Geometry: final body of the model. Coordinates: model frame, mm. A direction names the side the tool comes from. Coordinates: 2 decimals unless noted, no trailing zeros. Loops run counter-clockwise (first coordinate to the right, second up) from the corner with the lowest first, then second, coordinate; pieces in that order, holes last. Notation, with made-up numbers: (-31, 76.25) - (-11, 76.25) arc R14 cw to (-11, 82.25) - close; hole circle Ø1 at (-31.5, 79). An arc over 180 degrees is marked (long way). Answer in a Markdown table with one row per item.
from build123d import *

# Parameters (mm, degrees)
SKETCH1_W                                  = 115
SKETCH1_H                                  = 115
BOSS_EXTRUDE1_DEPTH                        = 40
FILLET1_R                                  = 10
SKETCH4_W                                  = 101
SKETCH4_H                                  = 101
CUT_EXTRUDE3_DEPTH                         = 40
SKETCH7_W                                  = 90
SKETCH7_H                                  = 90
CUT_EXTRUDE5_DEPTH                         = 60
FILLET3_R                                  = 10
SKETCH8_R                                  = 3.15
CUT_EXTRUDE6_DEPTH                         = 35
MIRROR2_AT_THE_SECOND_PLANE_COPY_1_SKETC_R = 3.15
MIRROR2_AT_THE_SECOND_PLANE_COPY_1_DEPTH   = 35
SKETCH9_R                                  = 1.25
CUT_EXTRUDE7_DEPTH                         = 15
MIRROR3_AT_THE_SECOND_PLANE_COPY_1_SKETC_R = 1.25
MIRROR3_AT_THE_SECOND_PLANE_COPY_1_DEPTH   = 15
SKETCH10_R                                 = 2.5
CUT_EXTRUDE8_DEPTH                         = 3
MIRROR4_AT_THE_SECOND_PLANE_COPY_1_SKETC_R = 2.5
MIRROR4_AT_THE_SECOND_PLANE_COPY_1_DEPTH   = 3
SKETCH11_W                                 = 40
SKETCH11_H                                 = 90
CUT_EXTRUDE9_DEPTH                         = 11
SKETCH13_W                                 = 2.5
SKETCH13_H                                 = 90
BOSS_EXTRUDE2_DEPTH                        = 17
FILLET6_R                                  = 2
SKETCH14_W                                 = 20
SKETCH14_H                                 = 30
CUT_EXTRUDE10_DEPTH                        = 11
SKETCH15_W                                 = 10
SKETCH15_H                                 = 2.5
BOSS_EXTRUDE3_DEPTH                        = 19
FILLET7_R                                  = 2
SKETCH16_W                                 = 115
SKETCH16_H                                 = 115
CUT_EXTRUDE12_DEPTH                        = 20
SKETCH17_W                                 = 10
SKETCH17_H                                 = 80
CUT_EXTRUDE13_DEPTH                        = 15
SKETCH20_R                                 = 2.25
CUT_EXTRUDE14_DEPTH                        = 25
MIRROR8_AT_THE_SECOND_PLANE_COPY_1_SKETC_R = 2.25
MIRROR8_AT_THE_SECOND_PLANE_COPY_1_DEPTH   = 25
SKETCH21_R                                 = 1.75
CUT_EXTRUDE15_DEPTH                        = 20
MIRROR9_AT_THE_SECOND_PLANE_COPY_1_SKETC_R = 1.75
MIRROR9_AT_THE_SECOND_PLANE_COPY_1_DEPTH   = 20
SKETCH24_W                                 = 15
SKETCH24_H                                 = 30
CUT_EXTRUDE16_DEPTH                        = 10
MIRROR10_AT_THE_SECOND_PLANE_COPY_1_SKET_W = 15
MIRROR10_AT_THE_SECOND_PLANE_COPY_1_SKET_H = 30
MIRROR10_AT_THE_SECOND_PLANE_COPY_1_DEPTH  = 10
SKETCH25_R                                 = 4
CUT_EXTRUDE17_DEPTH                        = 7.5
MIRROR11_AT_THE_SECOND_PLANE_COPY_1_SKET_R = 4
MIRROR11_AT_THE_SECOND_PLANE_COPY_1_DEPTH  = 7.5


with BuildPart() as part:
    # Sketch1 → Boss-Extrude1 (new, symmetric)
    with BuildSketch(Plane.XY):
        Rectangle(SKETCH1_W, SKETCH1_H)
    extrude(amount=BOSS_EXTRUDE1_DEPTH, both=True)

    # Fillet1
    fillet1_edges = [part.edges().sort_by_distance(p)[0] for p in [
        (-57.5, 57.5, 0),
        (57.5, 57.5, 0),
        (57.5, -57.5, 0),
        (-57.5, -57.5, 0),
    ]]
    fillet(fillet1_edges, radius=FILLET1_R)

    # Sketch4 → Cut-Extrude3 (cut)
    with BuildSketch(Plane.XY.offset(40)):
        Rectangle(SKETCH4_W, SKETCH4_H)
    extrude(amount=-CUT_EXTRUDE3_DEPTH, mode=Mode.SUBTRACT)

    # Sketch7 → Cut-Extrude5 (cut)
    with BuildSketch(Plane.XY):
        Rectangle(SKETCH7_W, SKETCH7_H)
    extrude(amount=-CUT_EXTRUDE5_DEPTH, mode=Mode.SUBTRACT)

    # Fillet3
    fillet3_edges = [part.edges().sort_by_distance(p)[0] for p in [
        (-45, -45, -20),
        (-45, 45, -20),
        (45, 45, -20),
        (45, -45, -20),
    ]]
    fillet(fillet3_edges, radius=FILLET3_R)

    # Sketch8 → Cut-Extrude6 (cut)
    with BuildSketch(Plane(origin=(0, 0, -40), x_dir=(-1, 0, 0), z_dir=(0, 0, -1))):
        with Locations((-48, 48)):
            Circle(SKETCH8_R)
    cut_extrude6 = extrude(amount=-CUT_EXTRUDE6_DEPTH, mode=Mode.SUBTRACT)

    # Mirror2: Cut-Extrude6 across plane
    add(cut_extrude6.mirror(Plane.ZX), mode=Mode.SUBTRACT)

    # Mirror2 at the second plane: Cut-Extrude6 across plane
    add(cut_extrude6.mirror(Plane(origin=(0, 0, 0), x_dir=(0, 0, 1), z_dir=(1, 0, 0))), mode=Mode.SUBTRACT)

    # Mirror2 at the second plane copy 1 sketc → Mirror2 at the second plane copy 1 (cut)
    with BuildSketch(Plane(origin=(0, 0, -40), x_dir=(1, 0, 0), z_dir=(0, 0, -1))):
        with Locations((-48, 48)):
            Circle(MIRROR2_AT_THE_SECOND_PLANE_COPY_1_SKETC_R)
    extrude(amount=-MIRROR2_AT_THE_SECOND_PLANE_COPY_1_DEPTH, mode=Mode.SUBTRACT)

    # Sketch9 → Cut-Extrude7 (cut)
    with BuildSketch(Plane.XY):
        with Locations((-48, 48)):
            Circle(SKETCH9_R)
    cut_extrude7 = extrude(amount=-CUT_EXTRUDE7_DEPTH, mode=Mode.SUBTRACT)

    # Mirror3: Cut-Extrude7 across plane
    add(cut_extrude7.mirror(Plane.ZX), mode=Mode.SUBTRACT)

    # Mirror3 at the second plane: Cut-Extrude7 across plane
    add(cut_extrude7.mirror(Plane(origin=(0, 0, 0), x_dir=(0, 0, 1), z_dir=(1, 0, 0))), mode=Mode.SUBTRACT)

    # Mirror3 at the second plane copy 1 sketc → Mirror3 at the second plane copy 1 (cut)
    with BuildSketch(Plane(origin=(0, 0, 0), x_dir=(-1, 0, 0), z_dir=(0, 0, 1))):
        with Locations((-48, 48)):
            Circle(MIRROR3_AT_THE_SECOND_PLANE_COPY_1_SKETC_R)
    extrude(amount=-MIRROR3_AT_THE_SECOND_PLANE_COPY_1_DEPTH, mode=Mode.SUBTRACT)

    # Sketch10 → Cut-Extrude8 (cut)
    with BuildSketch(Plane.XY):
        with Locations((-48, 48)):
            Circle(SKETCH10_R)
    cut_extrude8 = extrude(amount=-CUT_EXTRUDE8_DEPTH, mode=Mode.SUBTRACT)

    # Mirror4: Cut-Extrude8 across plane
    add(cut_extrude8.mirror(Plane.ZX), mode=Mode.SUBTRACT)

    # Mirror4 at the second plane: Cut-Extrude8 across plane
    add(cut_extrude8.mirror(Plane(origin=(0, 0, 0), x_dir=(0, 0, 1), z_dir=(1, 0, 0))), mode=Mode.SUBTRACT)

    # Mirror4 at the second plane copy 1 sketc → Mirror4 at the second plane copy 1 (cut)
    with BuildSketch(Plane(origin=(0, 0, 0), x_dir=(-1, 0, 0), z_dir=(0, 0, 1))):
        with Locations((-48, 48)):
            Circle(MIRROR4_AT_THE_SECOND_PLANE_COPY_1_SKETC_R)
    extrude(amount=-MIRROR4_AT_THE_SECOND_PLANE_COPY_1_DEPTH, mode=Mode.SUBTRACT)

    # Sketch11 → Cut-Extrude9 (cut)
    with BuildSketch(Plane(origin=(57.5, 0, 0), x_dir=(0, 0, -1), z_dir=(1, 0, 0))):
        with Locations((-40, 0)):
            Rectangle(SKETCH11_W, SKETCH11_H)
    extrude(amount=-CUT_EXTRUDE9_DEPTH, mode=Mode.SUBTRACT)

    # Sketch13 → Boss-Extrude2 (add)
    with BuildSketch(Plane(origin=(57.5, 0, 0), x_dir=(0, 0, -1), z_dir=(1, 0, 0))):
        with Locations((-18.75, 0)):
            Rectangle(SKETCH13_W, SKETCH13_H)
        Polygon((-17.5, -45), (-20, -45), (-40, -45), (-40, -47.5), (-17.5, -47.5), align=None)
        Polygon((-40, 45), (-20, 45), (-17.5, 45), (-17.5, 47.5), (-40, 47.5), align=None)
    extrude(amount=BOSS_EXTRUDE2_DEPTH)

    # Fillet6
    fillet6_edges = [part.edges().sort_by_distance(p)[0] for p in [
        (62.5, 45, 20),
        (62.5, -45, 20),
        (66, -47.5, 17.5),
        (66, 47.5, 17.5),
    ]]
    fillet(fillet6_edges, radius=FILLET6_R)

    # Sketch14 → Cut-Extrude10 (cut)
    with BuildSketch(Plane.ZY.offset(57.5)):
        with Locations((40, 0)):
            Rectangle(SKETCH14_W, SKETCH14_H)
    extrude(amount=-CUT_EXTRUDE10_DEPTH, mode=Mode.SUBTRACT)

    # Sketch15 → Boss-Extrude3 (add)
    with BuildSketch(Plane.ZY.offset(57.5)):
        Polygon((30, -15), (30, 15), (30, 17.5), (27.5, 17.5), (27.5, -17.5), (30, -17.5), align=None)
        with Locations((35, 16.25)):
            Rectangle(SKETCH15_W, SKETCH15_H)
        with Locations((35, -16.25)):
            Rectangle(SKETCH15_W, SKETCH15_H)
    extrude(amount=BOSS_EXTRUDE3_DEPTH)

    # Fillet7
    fillet7_edges = [part.edges().sort_by_distance(p)[0] for p in [
        (-63.5, -15, 30),
        (-63.5, 15, 30),
        (-67, 17.5, 27.5),
        (-67, -17.5, 27.5),
    ]]
    fillet(fillet7_edges, radius=FILLET7_R)

    # Sketch16 → Cut-Extrude12 (cut)
    with BuildSketch(Plane(origin=(0, 0, -40), x_dir=(-1, 0, 0), z_dir=(0, 0, -1))):
        Rectangle(SKETCH16_W, SKETCH16_H)
    extrude(amount=-CUT_EXTRUDE12_DEPTH, mode=Mode.SUBTRACT)

    # Sketch17 → Cut-Extrude13 (cut)
    with BuildSketch(Plane(origin=(0, 0, 17.5), x_dir=(-1, 0, 0), z_dir=(0, 0, -1))):
        with Locations((-62.5, 0)):
            Rectangle(SKETCH17_W, SKETCH17_H)
    extrude(amount=-CUT_EXTRUDE13_DEPTH, mode=Mode.SUBTRACT)

    # Sketch20 → Cut-Extrude14 (cut)
    with BuildSketch(Plane(origin=(57.5, 0, 0), x_dir=(0, 0, -1), z_dir=(1, 0, 0))):
        with Locations((10, 30)):
            Circle(SKETCH20_R)
    cut_extrude14 = extrude(amount=-CUT_EXTRUDE14_DEPTH, mode=Mode.SUBTRACT)

    # Mirror8: Cut-Extrude14 across plane
    add(cut_extrude14.mirror(Plane(origin=(0, 0, 0), x_dir=(0, 0, 1), z_dir=(1, 0, 0))), mode=Mode.SUBTRACT)

    # Mirror8 at the second plane: Cut-Extrude14 across plane
    add(cut_extrude14.mirror(Plane.ZX), mode=Mode.SUBTRACT)

    # Mirror8 at the second plane copy 1 sketc → Mirror8 at the second plane copy 1 (cut)
    with BuildSketch(Plane(origin=(-57.5, 0, 0), x_dir=(0, 0, -1), z_dir=(-1, 0, 0))):
        with Locations((10, 30)):
            Circle(MIRROR8_AT_THE_SECOND_PLANE_COPY_1_SKETC_R)
    extrude(amount=-MIRROR8_AT_THE_SECOND_PLANE_COPY_1_DEPTH, mode=Mode.SUBTRACT)

    # Sketch21 → Cut-Extrude15 (cut)
    with BuildSketch(Plane.XY.offset(40)):
        with Locations((30, 54)):
            Circle(SKETCH21_R)
    cut_extrude15 = extrude(amount=-CUT_EXTRUDE15_DEPTH, mode=Mode.SUBTRACT)

    # Mirror9: Cut-Extrude15 across plane
    add(cut_extrude15.mirror(Plane.ZX), mode=Mode.SUBTRACT)

    # Mirror9 at the second plane: Cut-Extrude15 across plane
    add(cut_extrude15.mirror(Plane(origin=(0, 0, 0), x_dir=(0, 0, 1), z_dir=(1, 0, 0))), mode=Mode.SUBTRACT)

    # Mirror9 at the second plane copy 1 sketc → Mirror9 at the second plane copy 1 (cut)
    with BuildSketch(Plane(origin=(0, 0, 40), x_dir=(-1, 0, 0), z_dir=(0, 0, 1))):
        with Locations((30, 54)):
            Circle(MIRROR9_AT_THE_SECOND_PLANE_COPY_1_SKETC_R)
    extrude(amount=-MIRROR9_AT_THE_SECOND_PLANE_COPY_1_DEPTH, mode=Mode.SUBTRACT)

    # Sketch24 → Cut-Extrude16 (cut)
    with BuildSketch(Plane(origin=(0, 57.5, 0), x_dir=(1, 0, 0), z_dir=(0, 1, 0))):
        with Locations((30, -20)):
            Rectangle(SKETCH24_W, SKETCH24_H)
    cut_extrude16 = extrude(amount=-CUT_EXTRUDE16_DEPTH, mode=Mode.SUBTRACT)

    # Mirror10: Cut-Extrude16 across plane
    add(cut_extrude16.mirror(Plane(origin=(0, 0, 0), x_dir=(0, 0, 1), z_dir=(1, 0, 0))), mode=Mode.SUBTRACT)

    # Mirror10 at the second plane: Cut-Extrude16 across plane
    add(cut_extrude16.mirror(Plane.ZX), mode=Mode.SUBTRACT)

    # Mirror10 at the second plane copy 1 sket → Mirror10 at the second plane copy 1 (cut)
    with BuildSketch(Plane(origin=(0, -57.5, 0), x_dir=(-1, 0, 0), z_dir=(0, -1, 0))):
        with Locations((30, -20)):
            Rectangle(MIRROR10_AT_THE_SECOND_PLANE_COPY_1_SKET_W, MIRROR10_AT_THE_SECOND_PLANE_COPY_1_SKET_H)
    extrude(amount=-MIRROR10_AT_THE_SECOND_PLANE_COPY_1_DEPTH, mode=Mode.SUBTRACT)

    # Sketch25 → Cut-Extrude17 (cut)
    with BuildSketch(Plane.ZY.offset(-45)):
        with Locations((-10, 30)):
            Circle(SKETCH25_R)
    cut_extrude17 = extrude(amount=-CUT_EXTRUDE17_DEPTH, mode=Mode.SUBTRACT)

    # Mirror11: Cut-Extrude17 across plane
    add(cut_extrude17.mirror(Plane.ZX), mode=Mode.SUBTRACT)

    # Mirror11 at the second plane: Cut-Extrude17 across plane
    add(cut_extrude17.mirror(Plane(origin=(0, 0, 0), x_dir=(0, 0, 1), z_dir=(1, 0, 0))), mode=Mode.SUBTRACT)

    # Mirror11 at the second plane copy 1 sket → Mirror11 at the second plane copy 1 (cut)
    with BuildSketch(Plane(origin=(-45, 0, 0), x_dir=(0, 0, 1), z_dir=(1, 0, 0))):
        with Locations((-10, 30)):
            Circle(MIRROR11_AT_THE_SECOND_PLANE_COPY_1_SKET_R)
    extrude(amount=-MIRROR11_AT_THE_SECOND_PLANE_COPY_1_DEPTH, mode=Mode.SUBTRACT)


solid = part.part
(1) Cut plane C-C on x = -5. Output: boundary loops of the cut face in (y, z).
Verdict:
| item | result |
|---|---|
| outline | (-57.5, -20) - (-45, -20) - (-45, 0) - (-50.5, 0) - (-50.5, 40) - (-57.5, 40) - close; (45, -20) - (57.5, -20) - (57.5, 40) - (50.5, 40) - (50.5, 0) - (45, 0) - close |
(2) Ray query, probe 1 along Y at (x, z) = (48, -2); probe 2 along X at (y, z) = (-21, 18); probe 3 along X at (y, z) = (-48, -12.25). Return the intervals inside material, ascending.
Verdict:
| item | result |
|---|---|
| probe 1 | y = -57.49 to -50.5, -45.5 to 45.5, 50.5 to 57.49 |
| probe 2 | x = -57.5 to -50.5, 50.5 to 57.5, 67.5 to 74.5 |
| probe 3 | x = -57.49 to -51.15, -44.85 to 44.85, 51.15 to 57.49 |
(3) First-contact query: pin 1 Ø9 at (y, z) = (30, -11) entering from +X; pin 2 Ø9 at (x, z) = (-69.5, 36.5) entering from -Y; pin 3 Ø13 at (x, y) = (-60.5, -2.5) entering from +Z. Flat tips, straight axial feed; report the tip coordinate or a pass-through.
Verdict:
| item | result |
|---|---|
| pin 1 | stops at x = 57.5 |
| pin 2 | stops at y = -17.5 |
| pin 3 | stops at z = 30 |
(4) Cut plane D-D on y = 30. State how many separate pieces and enclosed holes the cut face has, then the cut area to 4 significant figures.
Verdict:
| item | result |
|---|---|
| separate pieces | 5 |
| enclosed holes | 0 |
| area | 772.5 mm² |
(5) Cut plane B-B on x = -30. Output: boundary loops of the cut face in (y, z), then the cut area to 3 significant figures.
Verdict:
| item | result |
|---|---|
| outline | (-57.5, -20) - (-45, -20) - (-45, 0) - (-50.5, 0) - (-50.5, 5) - (-57.5, 5) - close; (-57.5, 35) - (-55.75, 35) - (-55.75, 40) - (-57.5, 40) - close; (-52.25, 35) - (-50.5, 35) - (-50.5, 40) - (-52.25, 40) - close; (45, -20) - (57.5, -20) - (57.5, 5) - (50.5, 5) - (50.5, 0) - (45, 0) - close; (50.5, 35) - (52.25, 35) - (52.25, 40) - (50.5, 40) - close; (55.75, 35) - (57.5, 35) - (57.5, 40) - (55.75, 40) - close |
| area | 605 mm² |
(6) Cut plane A-A on y = -7. Output: boundary loops of the cut face in (x, z), then the cut area to 3 significant figures.
Verdict:
| item | result |
|---|---|
| outline | (-76.5, 27.5) - (-57.5, 27.5) - (-57.5, -20) - (-45, -20) - (-45, 0) - (-50.5, 0) - (-50.5, 30) - (-76.5, 30) - close; (45, -20) - (57.5, -20) - (57.5, 20) - (50.5, 20) - (50.5, 0) - (45, 0) - close; (67.5, 17.5) - (74.5, 17.5) - (74.5, 20) - (67.5, 20) - close |
| area | 915 mm² |
(7) Access query for faces 5 (the face through (45.69, -47.04, -1.48)), 6 (the face through (-48.698, 33.966, -10.521)), 7 (the face through (-67, 17.5, 35)), 8 (the face through (-28, 54, 35)), 9 (the face through (-47, -47, -5)). Directions: +Z, -Z, +X, -X, +Y, -Y. A direction counts if a zero-diameter tool reaches every point of the face in a straight line with its end or side. Return the directions, or none.
Verdict:
| item | result |
|---|---|
| face 5 | +Z |
| face 6 | none |
| face 7 | +Z, -Z, -X, +Y |
| face 8 | +Y, -Y |
| face 9 | -Z |
(8) Pull-direction query (Z, two-part tool) for faces 1 (the face through (68, -1, 20)), 2 (the face through (70, -1, 17.5)), 3 (the face through (-45.69, -47.04, -1.48)), 4 (the face through (-55.035, 30.099, -7.752)); classes: pulls with the +Z half, pulls with the -Z half, needs draft (parallel to the pull), parting line crosses it, or undercut.
Verdict:
| item | result |
|---|---|
| face 1 | pulls with the +Z half |
| face 2 | pulls with the -Z half |
| face 3 | needs draft |
| face 4 | undercut |
